The listing builds one solid part. Answer for the finished solid, in the listing's coordinates (mm). Face numbers are marked on the shaded views. A direction names the side the tool comes from. Coordinates: 2 decimals unless noted, no trailing zeros. Loops run counter-clockwise (first coordinate to the right, second up) from the corner with the lowest first, then second, coordinate; pieces in that order, holes last. Notation, with made-up numbers: (61.25, 17) - (104.25, 17) arc R10 cw to (104.25, 22) - close; hole circle Ø3 at (51, 63). An arc over 180 degrees is marked (long way). Put each result on its own line as item: value.
```python
from build123d import *

# Parameters (mm, degrees)
SKETCH2_W           = 17.886691146
SKETCH2_H           = 2.175460001
CUT_EXTRUDE1_DEPTH  = 1.5
SKETCH3_W           = 6.296857424
SKETCH3_H           = 7.509086661
BOSS_EXTRUDE1_DEPTH = 3


with BuildPart() as part:
    # Sketch1 → Revolve1 (revolve)
    with BuildSketch(Plane(origin=(0, 0, 0), x_dir=(1, 0, 0), z_dir=(0, 1, 0))):
        Polygon((0, 0), (0, 10), (18.52566279, 10), (18.52566279, 6.890240487), (25.563295531, 6.890240487), (25.563295531, 4.677528689), (33.040780318, 4.677528689), (33.040780318, 8.152621406), (37.791182418, 8.152621406), (40.958117151, 5.953361174), (45.708519251, 5.953361174), (45.708519251, 0), align=None)
    revolve(axis=Axis((45.708519251, 0, 0), (-1, 0, 0)))

    # Sketch2 → Cut-Extrude1 (cut, symmetric)
    with BuildSketch(Plane(origin=(0, 0, 0), x_dir=(1, 0, 0), z_dir=(0, 1, 0))):
        with Locations((12.122244938, 9.650117441)):
            Rectangle(SKETCH2_W, SKETCH2_H)
        with Locations((12.122244938, -9.650117441)):
            Rectangle(SKETCH2_W, SKETCH2_H)
    extrude(amount=CUT_EXTRUDE1_DEPTH, both=True, mode=Mode.SUBTRACT)

    # Sketch3 → Boss-Extrude1 (add)
    with BuildSketch(Plane(origin=(45.708519251, 0, 0), x_dir=(0, 0, -1), z_dir=(1, 0, 0))):
        with Locations((-0.012160705, -0.001203589)):
            Rectangle(SKETCH3_W, SKETCH3_H)
    extrude(amount=BOSS_EXTRUDE1_DEPTH)


solid = part.part
```
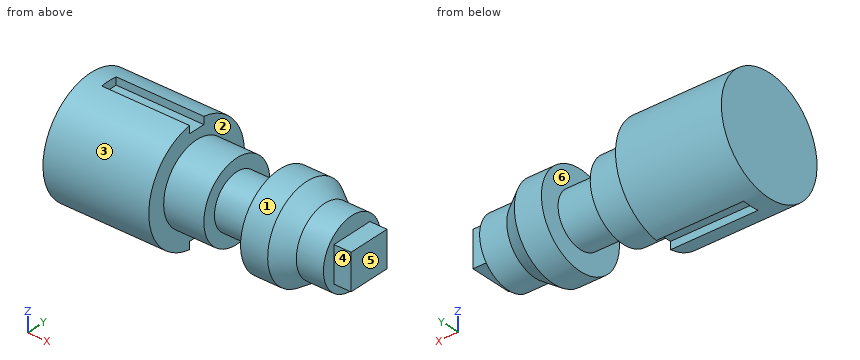
1) The part is cut by section A-A (x = 12.5). Give the vertices of the cut face in (y, z), and give its area (3 significant figures).
Found:
outline: (-1.5, -9.89) - (-1.5, -8.56) - (1.5, -8.56) - (1.5, -9.89) arc R10 ccw to (1.5, 9.89) - (1.5, 8.56) - (-1.5, 8.56) - (-1.5, 9.89) arc R10 ccw to start
area: 306 mm^2
2) For the marked faces 1, 2 and 3, determine the directions among +Z, -Z, +X, -X, +Y, -Y from which every point of the face is accessible in a straight line to the end or side of a thin tool.
Found:
face 1: +X
face 2: none
face 3: +X, -X
3) The part is cut by section D-D (x = 26.5). Give the vertices of the cut face in (y, z), and give its area (3 significant figures).
Found:
outline: circle Ø9.36 at (0, 0)
area: 68.7 mm^2
4) The part is cut by section C-C (z = 0). Give the vertices of the cut face in (x, y).
Found:
outline: (0, -10) - (18.53, -10) - (18.53, -6.89) - (25.56, -6.89) - (25.56, -4.68) - (33.04, -4.68) - (33.04, -8.15) - (37.79, -8.15) - (40.96, -5.95) - (45.71, -5.95) - (45.71, -3.76) - (48.71, -3.76) - (48.71, 3.75) - (45.71, 3.75) - (45.71, 5.95) - (40.96, 5.95) - (37.79, 8.15) - (33.04, 8.15) - (33.04, 4.68) - (25.56, 4.68) - (25.56, 6.89) - (18.53, 6.89) - (18.53, 10) - (0, 10) - close
5) The part is cut by section B-B (y = 0). Give the vertices of the cut face in (x, z), and give its area (3 significant figures).
Found:
outline: (0, -10) - (3.18, -10) - (3.18, -8.56) - (18.53, -8.56) - (18.53, -6.89) - (25.56, -6.89) - (25.56, -4.68) - (33.04, -4.68) - (33.04, -8.15) - (37.79, -8.15) - (40.96, -5.95) - (45.71, -5.95) - (45.71, -3.14) - (48.71, -3.14) - (48.71, 3.16) - (45.71, 3.16) - (45.71, 5.95) - (40.96, 5.95) - (37.79, 8.15) - (33.04, 8.15) - (33.04, 4.68) - (25.56, 4.68) - (25.56, 6.89) - (18.53, 6.89) - (18.53, 8.56) - (3.18, 8.56) - (3.18, 10) - (0, 10) - close
area: 691 mm^2
6) For a pull along X with two mould halves and no side action, classify the marked faces 4, 5 and 6 as pulls with the +X half, pulls with the -X half, needs draft (parallel to the pull), parting line crosses it, or undercut.
Found:
face 4: needs draft
face 5: pulls with the +X half
face 6: undercut
7) Straight lines are drawn through the part: L1, parallel to X at y = -2.5, z = -4; L2, parallel to X at y = 4.5, z = 8; L3, parallel to Y at x = 9, z = -1.5. For each, find the intervals that lie inside material, in ascending order. Write a range as [from, to].
Found:
L1: x = [0, 25.56], [33.04, 45.71]
L2: x = [0, 18.53]
L3: y = [-9.89, 9.89]
8) Each of these flat-tipped pins is pushed along its axis until it touches: pin 1 (1.5 mm diameter, centred on x = 46.5, y = -1.5, fed in from -Z); pin 2 (0.9 mm diameter, centred on x = 13.5, y = 0, fed in from +Z); pin 3 (5 mm diameter, centred on x = 13, z = -3.5, fed in from +Y). Where does it stop, or does it pass through?
Found:
pin 1: stops at z = -3.14
pin 2: stops at z = 8.56
pin 3: stops at y = 9.95
